CAD build for the part. Positions are in the model's coordinates, mm. Face numbers are marked on the shaded views. A direction names the side the tool comes from. Coordinates: 2 decimals unless noted, no trailing zeros. Order: outer loops, then holes, each group sorted by start corner. A loop starts at its lowest first (then second) coordinate and runs counter-clockwise, first axis right, second up. Notation, with made-up numbers: (88.25, -3.75) - (113.25, -3.75) arc R29 ccw to (113.25, 19.25) - close; hole circle Ø1 at (44.5, 34). An arc over 180 degrees is marked (long way). Write each question's results on one line, items separated by ' | '. Start each with the question number.
Q1. Band-saw the part on A-A, the plane y = 8.5. Write the cut outline in (x, z).
Q2. Pin check, flat tips, straight feed: P1, Ø12, axis at x = -76.2, z = 25.4, coming from the +Y side; P2, Ø2.5, axis at x = -50.8, y = 16.25, coming from the +Z side; P3, Ø2.5, axis at x = -26, z = -24, coming from the +Y side; P4, Ø1.5, axis at y = 45, z = -32.5, coming from the +X side. Stop position of each tip, or through.
Q3. Pull direction Z, two halves, no side cores. Call the marked faces 3, 4 and 5: released by +Z, released by -Z, zero draft, split by the parting line, or undercut.
Q4. Band-saw the part on B-B, the plane x = -76.2. Write the cut outline in (y, z), then the cut area to 3 significant figures.
Q5. Wall check: probe 1 along X at (y, z) = (4.6, -25.4); probe 2 along Z at (x, y) = (-76, 4); probe 3 along Y at (x, z) = (-50.8, -75). Give the ranges that are in metal, low to high.
Q6. Band-saw the part on C-C, the plane z = -8.5. Write the cut outline in (x, y), then the cut area to 3 significant figures.
Q7. Band-saw the part on D-D, the plane y = 35. Write the cut outline in (x, z), then the cut area to 3 significant figures.
Q8. Which spindle directions (+Z, -Z, +X, -X, +Y, -Y) get a long thin tool onto all of the face, cutting with end or side? Do the marked faces 1 and 2. Say none if no direction does.
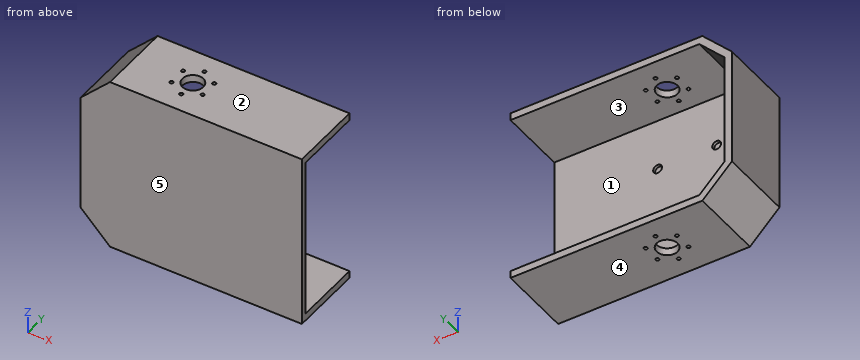
```python
from build123d import *

# Parameters (mm, degrees)
SKETCH2_W           = 190.5
SKETCH2_H           = 152.4
BOSS_EXTRUDE1_DEPTH = 5.08
CHAMFER1_SIZE       = 25.4
BOSS_EXTRUDE3_DEPTH = 58.42
SKETCH5_R           = 9
SKETCH5_R_2         = 1.5
CUT_EXTRUDE1_DEPTH  = 153.4
SKETCH7_R           = 3.81
CUT_EXTRUDE2_DEPTH  = 2.54


with BuildPart() as part:
    # Sketch2 → Boss-Extrude1 (new body)
    with BuildSketch(Plane(origin=(0, 0, 0), x_dir=(1, 0, 0), z_dir=(0, 1, 0))):
        with Locations((-31.75, 0)):
            Rectangle(SKETCH2_W, SKETCH2_H)
    extrude(amount=BOSS_EXTRUDE1_DEPTH)

    # Chamfer1
    chamfer1_edges = [part.edges().sort_by_distance(p)[0] for p in [
        (-127, 2.54, -76.2),
        (-127, 2.54, 76.2),
    ]]
    chamfer(chamfer1_edges, length=CHAMFER1_SIZE)

    # Sketch4 → Boss-Extrude3 (add)
    with BuildSketch(Plane(origin=(0, 5.08, 0), x_dir=(1, 0, 0), z_dir=(0, 1, 0))):
        Polygon((57.15, 69.85), (-98.969743879, 69.85), (-120.65, 48.169743879), (-120.65, -48.169743879), (-98.969743879, -69.85), (57.15, -69.85), (63.5, -69.85), (63.5, -76.2), (-101.6, -76.2), (-127, -50.8), (-127, 50.8), (-101.6, 76.2), (63.5, 76.2), (63.5, 69.85), align=None)
    extrude(amount=BOSS_EXTRUDE3_DEPTH)

    # Sketch5 → Cut-Extrude1 (cut, through all)
    with BuildSketch(Plane.XY.offset(76.2)):
        with Locations((-50.8, 31.75)):
            Circle(SKETCH5_R)
        with Locations((-50.8, 47.25)):
            Circle(SKETCH5_R_2)
        with Locations((-37.376606241, 39.5)):
            Circle(SKETCH5_R_2)
        with Locations((-37.376606241, 24)):
            Circle(SKETCH5_R_2)
        with Locations((-50.8, 16.25)):
            Circle(SKETCH5_R_2)
        with Locations((-64.223393759, 24)):
            Circle(SKETCH5_R_2)
        with Locations((-64.223393759, 39.5)):
            Circle(SKETCH5_R_2)
    extrude(amount=-CUT_EXTRUDE1_DEPTH, mode=Mode.SUBTRACT)

    # Sketch7 → Cut-Extrude2 (cut)
    with BuildSketch(Plane(origin=(0, 5.08, 0), x_dir=(1, 0, 0), z_dir=(0, 1, 0))):
        with Locations((-76.2, 25.4)):
            Circle(SKETCH7_R)
        with Locations((-25.4, 25.4)):
            Circle(SKETCH7_R)
        with Locations((-25.4, -25.4)):
            Circle(SKETCH7_R)
        with Locations((-76.2, -25.4)):
            Circle(SKETCH7_R)
    extrude(amount=-CUT_EXTRUDE2_DEPTH, mode=Mode.SUBTRACT)


solid = part.part
```
Results below:
1) outline: (-127, -50.8) - (-101.6, -76.2) - (63.5, -76.2) - (63.5, -69.85) - (-98.97, -69.85) - (-120.65, -48.17) - (-120.65, 48.17) - (-98.97, 69.85) - (63.5, 69.85) - (63.5, 76.2) - (-101.6, 76.2) - (-127, 50.8) - close
2) P1: stops at y = 5.08 | P2: passes through | P3: stops at y = 2.54 | P4: stops at x = -120.65
3) face 3: undercut | face 4: released by -Z | face 5: zero draft
4) outline: (0, -76.2) - (63.5, -76.2) - (63.5, -69.85) - (5.08, -69.85) - (5.08, -29.21) - (2.54, -29.21) - (2.54, -21.59) - (5.08, -21.59) - (5.08, 21.59) - (2.54, 21.59) - (2.54, 29.21) - (5.08, 29.21) - (5.08, 69.85) - (63.5, 69.85) - (63.5, 76.2) - (0, 76.2) - close | area: 1,480 mm²
5) probe 1: x = -127 to -80.01, -72.39 to -29.21, -21.59 to 63.5 | probe 2: z = -76.2 to -29.2, -21.6 to 21.6, 29.2 to 76.2 | probe 3: y = 0 to 14.75, 17.75 to 22.75, 40.75 to 45.75, 48.75 to 63.5
6) outline: (-127, 0) - (63.5, 0) - (63.5, 5.08) - (-120.65, 5.08) - (-120.65, 63.5) - (-127, 63.5) - close | area: 1,340 mm²
7) outline: (-127, -50.8) - (-101.6, -76.2) - (-59.19, -76.2) - (-59.19, -69.85) - (-98.97, -69.85) - (-120.65, -48.17) - (-120.65, 48.17) - (-98.97, 69.85) - (-59.19, 69.85) - (-59.19, 76.2) - (-101.6, 76.2) - (-127, 50.8) - close; (-42.41, -76.2) - (63.5, -76.2) - (63.5, -69.85) - (-42.41, -69.85) - close; (-42.41, 69.85) - (63.5, 69.85) - (63.5, 76.2) - (-42.41, 76.2) - close | area: 2,920 mm²
8) face 1: +X, +Y | face 2: +Z, +X, -X, +Y, -Y
